Verification items for the finished model (mm, model axes). Round coordinates to 2 decimals unless told otherwise and drop trailing zeros. Loops run counter-clockwise (first coordinate to the right, second up) from the corner with the lowest first, then second, coordinate; pieces in that order, holes last.
Autodesk Inventor part; units mm, degrees
ref_plane "YZ Plane" through (0, 0, 0) normal (1, 0, 0) x (0, 1, 0)
ref_plane "XZ Plane" through (0, 0, 0) normal (0, 1, 0) x (-1, 0, 0)
ref_plane "XY Plane" through (0, 0, 0) normal (0, 0, 1) x (1, 0, 0)
sketch "Esboço1" plane through (0, 0, 0) normal (0, 0, 1) x (1, 0, 0)
  line L0 (7.0711, 0) -> (422.9289, 0)
  line L1 (430, 7.0711) -> (430, 422.9289)
  line L2 (422.9289, 430) -> (7.0711, 430)
  line L3 (0, 422.9289) -> (0, 7.0711)
  line L4 (17.0711, 420) -> (412.9289, 420)
  line L5 (420, 412.9289) -> (420, 17.0711)
  line L6 (412.9289, 10) -> (17.0711, 10)
  line L7 (10, 17.0711) -> (10, 412.9289)
  line L8 (420, 17.0711) -> (222.0711, 215)
  line L9 (215, 222.0711) -> (17.0711, 420)
  line L10 (412.9289, 10) -> (215, 207.9289)
  line L11 (207.9289, 215) -> (10, 412.9289)
  line L12 (10, 17.0711) -> (207.9289, 215)
  line L13 (215, 222.0711) -> (412.9289, 420)
  line L14 (17.0711, 10) -> (215, 207.9289)
  line L15 (222.0711, 215) -> (420, 412.9289)
  line L16 (425.0292, 432.1003) -> (430.6066, 437.6777)
  line L17 (437.6777, 437.6777) -> (437.6777, 437.6777)
  line L18 (437.6777, 430.6066) -> (432.1421, 425.0711)
  line L19 (-2.1003, 425.0292) -> (-7.6777, 430.6066)
  line L20 (-7.6777, 437.6777) -> (-7.6777, 437.6777)
  line L21 (-0.6066, 437.6777) -> (4.9708, 432.1003)
  line L22 (4.9289, -2.1421) -> (-0.6066, -7.6777)
  line L23 (-7.6777, -7.6777) -> (-7.6777, -7.6777)
  line L24 (-7.6777, -0.6066) -> (-2.1003, 4.9708)
  line L25 (425.0711, -2.1421) -> (430.6066, -7.6777)
  line L26 (437.6777, -7.6777) -> (437.6777, -7.6777)
  line L27 (437.6777, -0.6066) -> (432.1421, 4.9289)
  arc A0 (437.6777, 430.6066) -> (437.6777, 437.6777) centre (434.1421, 434.1421) ccw
  arc A1 (437.6777, 437.6777) -> (430.6066, 437.6777) centre (434.1421, 434.1421) ccw
  arc A2 (-0.6066, 437.6777) -> (-7.6777, 437.6777) centre (-4.1421, 434.1421) ccw
  arc A3 (-7.6777, 437.6777) -> (-7.6777, 430.6066) centre (-4.1421, 434.1421) ccw
  arc A4 (-7.6777, -0.6066) -> (-7.6777, -7.6777) centre (-4.1421, -4.1421) ccw
  arc A5 (-7.6777, -7.6777) -> (-0.6066, -7.6777) centre (-4.1421, -4.1421) ccw
  arc A6 (430.6066, -7.6777) -> (437.6777, -7.6777) centre (434.1421, -4.1421) ccw
  arc A7 (437.6777, -7.6777) -> (437.6777, -0.6066) centre (434.1421, -4.1421) ccw
  circle A8 centre (-4.1421, 434.1421) radius 2
  circle A9 centre (434.1421, 434.1421) radius 2
  circle A10 centre (434.1421, -4.1421) radius 2
  circle A11 centre (-4.1421, -4.1421) radius 2
  line L28 (432.1421, 432.1003) -> (-2.1003, 432.1003)
  line L29 (-2.1003, 432.1003) -> (-2.1003, -2.1421)
  line L30 (-2.1003, -2.1421) -> (432.1421, -2.1421)
  line L31 (432.1421, -2.1421) -> (432.1421, 432.1003)
  line L32 (0, 0) -> (430, 0)
  line L33 (430, 0) -> (430, 430)
  line L34 (430, 430) -> (0, 430)
  line L35 (0, 430) -> (0, 0)
  point P0 (-7.6777, -7.6777)
  dimension "d2" = 10
  dimension "d11" = 5
  dimension "d12" = 4
  dimension "d13" = 4
  dimension "d14" = 4
  dimension "d15" = 4
extrude "Extrusão2" add sketch "Esboço1" along normal blind 15 contours L32 L35 L3 L34 L2 L33 L1 L0 | L16 A1 A0 L18 L31 L28 | L28 L29 L19 A3 A2 L21 | L27 A7 A6 L25 L30 L31 | L29 L30 L22 A5 A4 L24
extrude "Extrusão3" add sketch "Esboço1" along normal blind 15 and the other way blind 4 contours L28 L31 L30 L29
properties part number "base de calibração" material "MDF - Chapa de fibra de média densidade"
1. Release check for a two-part mould opening along Y. For faces 1 (the face through (214, 216, 0)), 2 (the face through (212, 420, 7)), 3 (the face through (432, 433.8, 0)), 4 (the face through (212, -2.142, 5)) record: released by +Y, released by -Y, zero draft, split by the parting line, or undercut.
2. Section check A-A (x = 26.5). Enter the section's corners in (y, z).
3. Gauge pin test, flat ends, axial feed: P1, Ø4, axis at x = 309.5, z = -1, coming from the -Y side; P2, Ø4.5, axis at y = 189, z = -2.5, coming from the -X side; P3, Ø4, axis at x = 431, y = -5, coming from the -Z side. Record the tip position at first contact, or that the pin passes through.
4. Section check B-B (y = 190). Enter the section's corners in (x, z), then the cut area to 3 significant figures.
5. Scan lines: L1, parallel to Y at x = 135, z = -1.25; L2, parallel to X at y = 166, z = -0.75; L3, parallel to Y at x = 213.5, z = 6.5. Record each from-to range of solid material in increasing order.
6. Section check C-C (z = 5.75). Give the number of separate pieces and of enclosed holes in the cut face, then the cut area to 3 significant figures.
Taken from the geometry:
1. face 1: undercut
1. face 2: undercut
1. face 3: zero draft
1. face 4: released by -Y
2. outline: (-2.14, -4) - (0, -4) - (0, 0) - (10, 0) - (10, 15) - (-2.14, 15) - close; (19.43, 0) - (33.57, 0) - (33.57, 15) - (19.43, 15) - close; (396.43, 0) - (410.57, 0) - (410.57, 15) - (396.43, 15) - close; (420, 0) - (430, 0) - (430, -4) - (432.1, -4) - (432.1, 15) - (420, 15) - close
3. P1: stops at y = -2.14
3. P2: stops at x = -2.1
3. P3: stops at z = 0
4. outline: (-2.1, -4) - (0, -4) - (0, 0) - (10, 0) - (10, 15) - (-2.1, 15) - close; (182.93, 0) - (197.07, 0) - (197.07, 15) - (182.93, 15) - close; (232.93, 0) - (247.07, 0) - (247.07, 15) - (232.93, 15) - close; (420, 0) - (430, 0) - (430, -4) - (432.14, -4) - (432.14, 15) - (420, 15) - close
4. area: 805 mm2
5. L1: y = -2.14 to 0, 430 to 432.1
5. L2: x = -2.1 to 0, 430 to 432.14
5. L3: y = -2.14 to 10, 206.43 to 223.57, 420 to 432.1
6. separate pieces: 1
6. enclosed holes: 8
6. area: 32,200 mm2
